from build123d import *

# Parameters (mm, degrees)
EXTRUDE1_DEPTH     = 12.7
SKETCH3_R          = 3.1115
CUT_EXTRUDE1_DEPTH = 12.7


with BuildPart() as part:
    # Sketch2 → Extrude1 (new body)
    with BuildSketch(Plane.XY):
        with BuildLine():
            Line((10375.902142089, 13017.500110193), (10375.902142089, 13102.653009206))
            ThreePointArc((10375.902142089, 13102.653009206), (10374.042270149, 13107.143137266), (10369.552142089, 13109.003009206))
            Line((10369.552142089, 13109.003009206), (10337.802142089, 13109.003009206))
            Line((10337.802142089, 13109.003009206), (10337.800747814, 14185.900110193))
            Line((10337.800747814, 14185.900110193), (10852.147924282, 14185.900110193))
            Line((10852.147924282, 14185.900110193), (10852.150747814, 13123.290509206))
            Line((10852.150747814, 13123.290509206), (10823.581236416, 13123.290509206))
            Line((10823.581236416, 13123.290509206), (10823.581236416, 13165.835509206))
            ThreePointArc((10823.581236416, 13165.835509206), (10821.295236416, 13168.121509206), (10819.009236416, 13165.835509206))
            Line((10819.009236416, 13165.835509206), (10819.009236416, 13123.290509206))
            Line((10819.009236416, 13123.290509206), (10804.525747814, 13123.290509206))
            ThreePointArc((10804.525747814, 13123.290509206), (10798.175747814, 13116.940509206), (10804.525747814, 13110.590509206))
            Line((10804.525747814, 13110.590509206), (10804.525747814, 13017.500110193))
            Line((10804.525747814, 13017.500110193), (10616.625223517, 13017.500110193))
            Line((10616.625223517, 13017.500110193), (10559.649893716, 13085.667043341))
            ThreePointArc((10559.649893716, 13085.667043341), (10557.466824452, 13087.347190416), (10554.77765388, 13087.944724716))
            Line((10554.77765388, 13087.944724716), (10467.552782059, 13087.944724716))
            ThreePointArc((10467.552782059, 13087.944724716), (10463.062653998, 13086.084852777), (10461.202782059, 13081.594724716))
            Line((10461.202782059, 13081.594724716), (10461.202782059, 13017.500110193))
            Line((10461.202782059, 13017.500110193), (10375.902142089, 13017.500110193))
        make_face()
    extrude(amount=-EXTRUDE1_DEPTH)

    # Sketch3 → Cut-Extrude1 (cut)
    with BuildSketch(Plane.XY):
        with Locations((10387.012550678, 13062.712110193)):
            Circle(SKETCH3_R)
        with Locations((10387.012550678, 13037.312110193)):
            Circle(SKETCH3_R)
        with Locations((10788.650050678, 13062.712110193)):
            Circle(SKETCH3_R)
        with Locations((10788.650050678, 13037.312110193)):
            Circle(SKETCH3_R)
    extrude(amount=-CUT_EXTRUDE1_DEPTH, mode=Mode.SUBTRACT)


solid = part.part
Geometry: final body of the model. Coordinates: model frame, mm. A direction names the side the tool comes from. Round coordinates to 2 decimals unless told otherwise and drop trailing zeros. Loops run counter-clockwise (first coordinate to the right, second up) from the corner with the lowest first, then second, coordinate; pieces in that order, holes last. Notation, with made-up numbers: (-14, 81.5) -> (-8, 81.5) arc R9 cw to (-8, 92.5) -> close; hole circle Ø3 at (40.25, 23.5). An arc over 180 degrees is marked (long way). One line per question, with ' | ' between items. Start each with the question number.
1. Section B-B on x = 10498. Output: boundary loops of the cut face in (y, z).
2. Set-up query: faces 1 (the face through (10588.536, 13051.106, -6.261)), 2 (the face through (10599, 13610, -12.7)). Return all of +Z, -Z, +X, -X, +Y, -Y with unobstructed straight access to the full face (end or side cutting, diameter ignored); none if empty.
3. Section A-A on z = -7.75. Output: boundary loops of the cut face in (x, y).
4. Line query: line 1 along Y through (x, z) = (10535.5, -3); line 2 along X through (y, z) = (14106.5, -8.75); line 3 along Y through (x, z) = (10815, -2). Output: solid intervals per line, ascending. Write a range as [from, to].
Returned:
1) outline: (13087.94, -12.7) -> (14185.9, -12.7) -> (14185.9, 0) -> (13087.94, 0) -> close
2) face 1: +Z, -Z, -Y | face 2: -Z, +X, -X, +Y, -Y
3) outline: (10337.8, 13109) -> (10369.55, 13109) arc R6.35 cw to (10375.9, 13102.65) -> (10375.9, 13017.5) -> (10461.2, 13017.5) -> (10461.2, 13081.59) arc R6.35 cw to (10467.55, 13087.94) -> (10554.78, 13087.94) arc R6.35 cw to (10559.65, 13085.67) -> (10616.63, 13017.5) -> (10804.53, 13017.5) -> (10804.53, 13110.59) arc R6.35 cw to (10804.53, 13123.29) -> (10819.01, 13123.29) -> (10819.01, 13165.84) arc R2.29 cw to (10823.58, 13165.84) -> (10823.58, 13123.29) -> (10852.15, 13123.29) -> (10852.15, 14185.9) -> (10337.8, 14185.9) -> close; hole circle Ø6.22 at (10387.01, 13037.31); hole circle Ø6.22 at (10387.01, 13062.71); hole circle Ø6.22 at (10788.65, 13037.31); hole circle Ø6.22 at (10788.65, 13062.71)
4) line 1: y = [13087.94, 14185.9] | line 2: x = [10337.8, 10852.15] | line 3: y = [13123.29, 14185.9]
